```python
from build123d import *

# Parameters (mm, degrees)
F1_W           = 600
F1_H           = 1000
F2_DEPTH       = 28
F3_R           = 10
F5_D           = 8.2
F5_DEPTH       = 20
F5_CBORE_D     = 20
F5_CBORE_DEPTH = 11
F5_TIP         = 2.463528538


with BuildPart() as f2:
    # F1 (on offset) → F2 (new body)
    with BuildSketch(Plane.XY.offset(850)):
        Rectangle(F1_W, F1_H)
    extrude(amount=F2_DEPTH)

    # F3
    f3_edges = [f2.edges().sort_by_distance(p)[0] for p in [
        (300, 0, 878),
    ]]
    fillet(f3_edges, radius=F3_R)

    # F5
    with Locations(Plane(origin=(0, 0, 850), x_dir=(1, 0, 0), z_dir=(0, 0, -1))):
        with Locations((250, 325), (250, -305), (-250, -305), (-250, 325)):
            CounterBoreHole(F5_D / 2, F5_CBORE_D / 2, F5_CBORE_DEPTH, depth=F5_DEPTH)
            with Locations((0, 0, -(F5_DEPTH + F5_TIP / 2))):  # 118° drill point
                Cone(0, F5_D / 2, F5_TIP, mode=Mode.SUBTRACT)


solid = f2.part
```
Verification items for the finished model (mm, model axes). A direction names the side the tool comes from. Round coordinates to 2 decimals unless told otherwise and drop trailing zeros. Answer as a JSON object with one key per item and string values. Group by question number.
Q1. Mould release check, pull along X, two halves, no side actions. Record for faces 1 (the flat face through (-300, -7, 864)), 2 (the flat face through (249.9, 309.3, 861)), 3 (the flat face through (-4, -500, 864)), 4 (the cylindrical face through (-240.763, 308.83, 855.423)): released by +X, released by -X, zero draft, split by the parting line, or undercut.
Q2. Thickness scan on line 1 (Y direction, x = 250, z = 865); line 2 (X direction, y = -325, z = 866.5); line 3 (X direction, y = -325, z = 856.5). Record the ranges inside material, lowest first.
Q3. Go/stop test with flat-tipped pins: pin 1 Ø22 at (x, y) = (247.5, -322.5) entering from -Z; pin 2 Ø13 at (x, y) = (-250, -325) entering from -Z; pin 3 Ø6 at (y, z) = (6.5, 871.5) entering from +X. Record where each tip stops, or that it passes through.
Q4. Tool access check on faces 5 (the flat face through (-4, 500, 864)), 6 (the cylindrical face through (259.54, -328, 855.42)). Record the directions out of +Z, -Z, +X, -X, +Y, -Y that give a thin tool (end or side, any length) a straight path to the whole face; none if there is none.
Found:
{
 "1": {"face 1": "released by -X", "face 2": "undercut", "face 3": "zero draft", "face 4": "undercut"},
 "2": {"line 1": "y = -500 to -329.1, -320.9 to 300.9, 309.1 to 500", "line 2": "x = -300 to -254.1, -245.9 to 245.9, 254.1 to 300", "line 3": "x = -300 to -260, -240 to 240, 260 to 300"},
 "3": {"pin 1": "stops at z = 850", "pin 2": "stops at z = 861", "pin 3": "stops at x = 299.99"},
 "4": {"face 5": "+Z, -Z, +X, -X, +Y", "face 6": "-Z"}
}
